Input: part model. Units: mm. Frame: model coordinates. A direction names the side the tool comes from. Give positions to 0.01 mm unless a question says otherwise; leave off trailing zeros. Loops run counter-clockwise (first coordinate to the right, second up) from the corner with the lowest first, then second, coordinate; pieces in that order, holes last. Notation, with made-up numbers: M 31.5,81 L 47.5,81 A20 ccw 47.5,109 Z; hole C -25.75,-22 d6. An arc over 180 degrees is marked long. Answer as a JSON object with one key per item and string values. Group by question number.
1) Access query for faces 1 (the flat face through (89, 5, -76.2)), 2 (the cylindrical face through (60.95, 4.7, -63.39)), 3 (the flat face through (13, 5, -76.2)). Directions: +Z, -Z, +X, -X, +Y, -Y. A direction counts if a zero-diameter tool reaches every point of the face in a straight line with its end or side. Return the directions, or none.
2) Section query A-A on z = -38.1. Return loops of the section in (x, y) (3 decimals).
3) Section query D-D on x = 50.8. Return loops of the section in (y, z) (3 decimals).
4) First-contact query: P1, Ø2, axis at y = 6, z = -102.5, coming from the -X side; P2, Ø3, axis at x = 92, y = 3, coming from the -Z side; P3, Ø4, axis at y = 5.5, z = -93, coming from the +X side. Flat tips, straight axial feed; report the tip coordinate or a pass-through.
5) Draft query along X for faces 4 (the cylindrical face through (39.278, 4.696, -65.765)), 5 (the flat face through (25.4, 5, -101)), 6 (the flat face through (101.6, 5, -38)), 7 (the flat face through (50, 0, -50)). Return one class per face: +X half, -X half, draft (parallel to the pull), parting line (faces both ways), or undercut.
6) Section query B-B on x = 88.9. Return loops of the section in (y, z) (3 decimals), plus the area to 3 significant figures.
7) Ray query, L1, parallel to Z at x = 12.7, y = 2.75; L2, parallel to X at y = 3.75, z = -11; L3, parallel to Z at x = 87, y = 5.25. Return the intervals inside material, ascending.
8) Section query C-C on z = -78. Return loops of the section in (x, y) (3 decimals).
from build123d import *

# Parameters (mm, degrees)
SKETCH1_W                   = 101.6
SKETCH1_H                   = 127
BOSS_EXTRUDE1_DEPTH         = 9.525
SKETCH2_R                   = 17.018
CUT_EXTRUDE1_DEPTH          = 10.525
F_1_4_CLEARANCE_HOLE1_D     = 6.7564
LPATTERN1_COUNT             = 2
LPATTERN1_PITCH             = 25.4
LPATTERN1_COUNT_DIR2        = 4
LPATTERN1_PITCH_DIR2        = 25.4
TAP_DRILL_FOR_1_4_20_TAP1_D = 5.1054
LPATTERN2_COUNT             = 4
LPATTERN2_PITCH             = 25.4
SKETCH7_W                   = 25.4
SKETCH7_H                   = 50.8
CUT_EXTRUDE2_DEPTH          = 10.525
LPATTERN3_COUNT             = 2
LPATTERN3_PITCH             = 42.291


with BuildPart() as part:
    # Sketch1 → Boss-Extrude1 (new body)
    with BuildSketch(Plane(origin=(0, 0, 0), x_dir=(1, 0, 0), z_dir=(0, 1, 0))):
        with Locations((50.8, 63.5)):
            Rectangle(SKETCH1_W, SKETCH1_H)
    extrude(amount=BOSS_EXTRUDE1_DEPTH)

    # Sketch2 → Cut-Extrude1 (cut, through all)
    with BuildSketch(Plane(origin=(0, 9.525, 0), x_dir=(1, 0, 0), z_dir=(0, 1, 0))):
        with Locations((50.8, 127)):
            Circle(SKETCH2_R)
    extrude(amount=-CUT_EXTRUDE1_DEPTH, mode=Mode.SUBTRACT)

    # 1/4 Clearance Hole1 (through all)
    with Locations(Plane(origin=(0, 9.525, 0), x_dir=(-1, 0, 0), z_dir=(0, 1, 0))):
        with Locations((-12.7, -12.7)):
            f_1_4_clearance_hole1 = Hole(F_1_4_CLEARANCE_HOLE1_D / 2)

    # LPattern1: 1_4 Clearance Hole1 2 × 4
    with Locations(*[(j * LPATTERN1_PITCH_DIR2, 0, -i * LPATTERN1_PITCH) for i in range(LPATTERN1_COUNT) for j in range(LPATTERN1_COUNT_DIR2) if (i, j) != (0, 0)]):
        add(f_1_4_clearance_hole1, mode=Mode.SUBTRACT)

    # Tap Drill for 1/4-20 Tap1 (through all)
    with Locations(Plane(origin=(0, 9.525, 0), x_dir=(-1, 0, 0), z_dir=(0, 1, 0))):
        with Locations((-12.7, -63.5)):
            tap_drill_for_1_4_20_tap1 = Hole(TAP_DRILL_FOR_1_4_20_TAP1_D / 2)

    # LPattern2: Tap Drill for 1/4-20 Tap1 ×4
    with Locations(*[(i * LPATTERN2_PITCH, 0, 0) for i in range(1, LPATTERN2_COUNT)]):
        add(tap_drill_for_1_4_20_tap1, mode=Mode.SUBTRACT)

    # Sketch7 → Cut-Extrude2 (cut, through all)
    with BuildSketch(Plane(origin=(0, 9.525, 0), x_dir=(1, 0, 0), z_dir=(0, 1, 0))):
        with Locations((12.7, 101.6)):
            Rectangle(SKETCH7_W, SKETCH7_H)
        with Locations((88.9, 101.6)):
            Rectangle(SKETCH7_W, SKETCH7_H)
    extrude(amount=-CUT_EXTRUDE2_DEPTH, mode=Mode.SUBTRACT)

    # Sketch8 → #8-32 Tapped Hole1 (revolve, cut)
    with BuildSketch(Plane(origin=(29.6545, 4.7625, -127), x_dir=(0, 1, 0), z_dir=(1, 0, 0))):
        Polygon((0, 0), (0, 11.705806461), (1.7272, 10.668), (1.7272, 0), align=None)
    f_8_32_tapped_hole1 = revolve(axis=Axis((29.6545, 4.7625, -133.35), (0, 0, 1)), mode=Mode.SUBTRACT)

    # LPattern3: #8-32 Tapped Hole1 ×2
    with Locations(*[(i * LPATTERN3_PITCH, 0, 0) for i in range(1, LPATTERN3_COUNT)]):
        add(f_8_32_tapped_hole1, mode=Mode.SUBTRACT)


solid = part.part
Output:
{
 "1": {"face 1": "-Z, +X, +Y, -Y", "face 2": "+Y, -Y", "face 3": "-Z, -X, +Y, -Y"},
 "2": {"outline": "M 0,0 L 9.322,0 L 9.322,9.525 L 0,9.525 Z; M 16.078,0 L 34.722,0 L 34.722,9.525 L 16.078,9.525 Z; M 41.478,0 L 60.122,0 L 60.122,9.525 L 41.478,9.525 Z; M 66.878,0 L 85.522,0 L 85.522,9.525 L 66.878,9.525 Z; M 92.278,0 L 101.6,0 L 101.6,9.525 L 92.278,9.525 Z"},
 "3": {"outline": "M 0,-109.982 L 9.525,-109.982 L 9.525,0 L 0,0 Z"},
 "4": {"P1": "stops at x = 25.4", "P2": "stops at z = -76.2", "P3": "stops at x = 76.2"},
 "5": {"face 4": "undercut", "face 5": "-X half", "face 6": "+X half", "face 7": "draft"},
 "6": {"outline": "M 0,-76.2 L 9.525,-76.2 L 9.525,-66.053 L 0,-66.053 Z; M 0,-60.947 L 9.525,-60.947 L 9.525,-41.478 L 0,-41.478 Z; M 0,-34.722 L 9.525,-34.722 L 9.525,-16.078 L 0,-16.078 Z; M 0,-9.322 L 9.525,-9.322 L 9.525,0 L 0,0 Z", "area": "548 mm^2"},
 "7": {"L1": "z = -76.2 to -66.05, -60.95 to -41.48, -34.72 to -16.08, -9.32 to 0", "L2": "x = 0 to 9.78, 15.62 to 35.18, 41.02 to 60.58, 66.42 to 85.98, 91.82 to 101.6", "L3": "z = -76.2 to -65.2, -61.8 to -40.89, -35.31 to -15.49, -9.91 to 0"},
 "8": {"outline": "M 25.4,0 L 76.2,0 L 76.2,9.525 L 25.4,9.525 Z"}
}
